from build123d import *

# Parameters (mm, degrees)
ESTRUSIONE_ESTRUSIONE1_DEPTH = 7


with BuildPart() as part:
    # Schizzo1 → Rivoluzione1 (revolve)
    with BuildSketch(Plane.XY, mode=Mode.PRIVATE) as rivoluzione1_sk:
        Polygon((0, 6), (0, 10.5), (13.5, 10.5), (13.5, 11), (20.5, 11), (20.5, 10.5), (34, 10.5), (34, 6), align=None)
    revolve(rivoluzione1_sk.sketch.rotate(Axis((0, 0, 0), (1, 0, 0)), 90), axis=Axis((0, 0, 0), (1, 0, 0)))

    # Schizzo2 → Estrusione-Estrusione1 (add)
    with BuildSketch(Plane(origin=(20.5, 0, 0), x_dir=(0, 0, -1), z_dir=(1, 0, 0))):
        with BuildLine():
            Line((-9.526279218, 5.500000386), (-12.701705922, 0))
            Line((-12.701705922, 0), (-9.526279182, -5.50000045))
            ThreePointArc((-9.526279182, -5.50000045), (-11, -3.7e-08), (-9.526279218, 5.500000386))
        make_face()
        with BuildLine():
            Line((-6.350852961, 11), (-9.526279218, 5.500000386))
            ThreePointArc((-9.526279218, 5.500000386), (-5.499999807, 9.526279553), (0, 11))
            Line((0, 11), (-6.350852961, 11))
        make_face()
        with BuildLine():
            Line((6.350852961, 11), (0, 11))
            ThreePointArc((0, 11), (5.499999692, 9.526279619), (9.526279086, 5.500000616))
            Line((9.526279086, 5.500000616), (6.350852961, 11))
        make_face()
        with BuildLine():
            ThreePointArc((0, -11), (-5.499999775, -9.526279572), (-9.526279182, -5.50000045))
            Line((-9.526279182, -5.50000045), (-6.350852961, -11))
            Line((-6.350852961, -11), (0, -11))
        make_face()
        with BuildLine():
            ThreePointArc((9.526279182, -5.50000045), (5.499999775, -9.526279572), (0, -11))
            Line((0, -11), (6.350852961, -11))
            Line((6.350852961, -11), (9.526279182, -5.50000045))
        make_face()
        with BuildLine():
            ThreePointArc((11, 0), (10.625184022, -2.847009747), (9.526279182, -5.50000045))
            Line((9.526279182, -5.50000045), (12.701705922, 0))
            Line((12.701705922, 0), (9.526279086, 5.500000616))
            ThreePointArc((9.526279086, 5.500000616), (10.625183997, 2.84700984), (11, 0))
        make_face()
    extrude(amount=-ESTRUSIONE_ESTRUSIONE1_DEPTH)


solid = part.part
The model under review builds one solid part; all positions refer to its coordinate system, in mm. A direction names the side the tool comes from. Round coordinates to 2 decimals unless told otherwise and drop trailing zeros. Loops run counter-clockwise (first coordinate to the right, second up) from the corner with the lowest first, then second, coordinate; pieces in that order, holes last. Notation, with made-up numbers: (59, 84.5) -> (85, 84.5) arc R20 ccw to (85, 109.5) -> close; hole circle Ø9 at (78.25, 51). An arc over 180 degrees is marked (long way). One line per question, with ' | ' between items. Start each with the question number.
Item 1: Add section D-D, the plane y = -9.5. Write out the cut boundary in (x, z), then the cut area to 3 significant figures.
Item 2: Add section A-A, the plane z = 0. Write out the cut boundary in (x, y).
Item 3: Add section B-B, the plane y = 2.75. Write out the cut boundary in (x, z), then the cut area to 3 significant figures.
Item 4: For pin 1 (8 mm diameter, centred on x = 8, y = -2, fed in from +Z); pin 2 (1.5 mm diameter, centred on x = 4, y = -3.5, fed in from +Z); pin 3 (1 mm diameter, centred on x = 23, y = 3, fed in from -Z), all flat-tipped, find the tip position at first contact; note any pin that passes through.
Item 5: Draft analysis for pull direction Z (two halves, no side actions). For faces 1 (the face through (13.5, -3.2, -10.3)), 2 (the face through (27.3, -3.2, 10)), 3 (the face through (16.762, -1.802, 5.723)), state which applies: +Z half, -Z half, draft (parallel to the pull), parting line (faces both ways), or undercut.
Item 6: Machinability: for faces 4 (the face through (17, 11, 0)), 5 (the face through (20.5, -3.2, -10.3)), 6 (the face through (6.8, -3.2, 10)), which of the approach directions +Z, -Z, +X, -X, +Y, -Y give a long, thin tool a straight path to every point of the face, cutting with its end or side? Answer none if there is none.
Item 7: Add section C-C, the plane x = 20. Write out the cut boundary in (y, z).
Item 8: Wall thickness on line 1 along Y through (x, z) = (21, 0); line 2 along Y through (x, z) = (4.5, 3.5); line 3 along Z through (x, y) = (18.5, 4): over which ranges is each line inside the solid? List them lowest first. Write a range as [from, to].
Return value:
1) outline: (0, -4.47) -> (13.5, -4.47) -> (13.5, -7.22) -> (20.5, -7.22) -> (20.5, -4.47) -> (34, -4.47) -> (34, 4.47) -> (20.5, 4.47) -> (20.5, 7.22) -> (13.5, 7.22) -> (13.5, 4.47) -> (0, 4.47) -> close | area: 343 mm2
2) outline: (0, -10.5) -> (13.5, -10.5) -> (13.5, -11) -> (20.5, -11) -> (20.5, -10.5) -> (34, -10.5) -> (34, -6) -> (0, -6) -> close; (0, 6) -> (34, 6) -> (34, 10.5) -> (20.5, 10.5) -> (20.5, 11) -> (13.5, 11) -> (13.5, 10.5) -> (0, 10.5) -> close
3) outline: (0, -10.13) -> (13.5, -10.13) -> (13.5, -11.11) -> (20.5, -11.11) -> (20.5, -10.13) -> (34, -10.13) -> (34, -5.33) -> (0, -5.33) -> close; (0, 5.33) -> (34, 5.33) -> (34, 10.13) -> (20.5, 10.13) -> (20.5, 11.11) -> (13.5, 11.11) -> (13.5, 10.13) -> (0, 10.13) -> close | area: 340 mm2
4) pin 1: stops at z = 10.5 | pin 2: stops at z = 10.13 | pin 3: stops at z = -10.2
5) face 1: draft | face 2: parting line | face 3: undercut
6) face 4: +Z, -Z, +X, -X, +Y | face 5: +X | face 6: -X
7) outline: (-11, -6.35) -> (0, -12.7) -> (11, -6.35) -> (11, 6.35) -> (0, 12.7) -> (-11, 6.35) -> close; hole circle Ø12 at (0, 0)
8) line 1: y = [-10.5, -6], [6, 10.5] | line 2: y = [-9.9, -4.87], [4.87, 9.9] | line 3: z = [-10.39, -4.47], [4.47, 10.39]
